Geometry check sheet. Reference: the model listing, model coordinates, mm. A direction names the side the tool comes from. Give positions to 0.01 mm unless a question says otherwise; leave off trailing zeros. Loops run counter-clockwise (first coordinate to the right, second up) from the corner with the lowest first, then second, coordinate; pieces in that order, holes last. Notation, with made-up numbers: (21.5, 76.25) -> (75.5, 76.25) arc R36 ccw to (75.5, 114.25) -> close; hole circle Ø9 at (-35, 72). An arc over 180 degrees is marked (long way). Answer as a JSON object with one key per item and string values.
from build123d import *

# Parameters (mm, degrees)
CROQUIS1_W              = 92
CROQUIS1_H              = 62
SALIENTE_EXTRUIR1_DEPTH = 18
CROQUIS2_W              = 87
CROQUIS2_H              = 57
CORTAR_EXTRUIR1_DEPTH   = 16
CROQUIS3_W              = 89
CROQUIS3_H              = 59
CROQUIS3_W_2            = 87
CROQUIS3_H_2            = 57
SALIENTE_EXTRUIR2_DEPTH = 2
CROQUIS4_W              = 2.5
CROQUIS4_H              = 14.150072655
CROQUIS4_H_2            = 13.999979608
CROQUIS4_H_3            = 17.009234147
CORTAR_EXTRUIR2_DEPTH   = 16
CROQUIS5_W              = 9.965409089
CROQUIS5_H              = 2.5
CROQUIS5_W_2            = 7.304626576
CROQUIS5_W_3            = 7.420347284
CROQUIS5_W_4            = 5
CORTAR_EXTRUIR3_DEPTH   = 5
CROQUIS7_R              = 2.5
CORTAR_EXTRUIR4_DEPTH   = 2
CROQUIS8_W              = 50.384335714
CROQUIS8_H              = 5
CORTAR_EXTRUIR5_DEPTH   = 2.5
CROQUIS9_W              = 56.605701511
CROQUIS9_H              = 16
CORTAR_EXTRUIR6_DEPTH   = 2.5


with BuildPart() as part:
    # Croquis1 → Saliente-Extruir1 (new body)
    with BuildSketch(Plane(origin=(0, 0, 0), x_dir=(1, 0, 0), z_dir=(0, 1, 0))):
        Rectangle(CROQUIS1_W, CROQUIS1_H)
    extrude(amount=SALIENTE_EXTRUIR1_DEPTH)

    # Croquis2 → Cortar-Extruir1 (cut)
    with BuildSketch(Plane(origin=(0, 18, 0), x_dir=(1, 0, 0), z_dir=(0, 1, 0))):
        Rectangle(CROQUIS2_W, CROQUIS2_H)
    extrude(amount=-CORTAR_EXTRUIR1_DEPTH, mode=Mode.SUBTRACT)

    # Croquis3 → Saliente-Extruir2 (add)
    with BuildSketch(Plane(origin=(0, 18, 0), x_dir=(1, 0, 0), z_dir=(0, 1, 0))):
        Rectangle(CROQUIS3_W, CROQUIS3_H)
        Rectangle(CROQUIS3_W_2, CROQUIS3_H_2, mode=Mode.SUBTRACT)
    extrude(amount=SALIENTE_EXTRUIR2_DEPTH)

    # Croquis4 → Cortar-Extruir2 (cut)
    with BuildSketch(Plane(origin=(0, 20, 0), x_dir=(1, 0, 0), z_dir=(0, 1, 0))):
        with Locations((-44.75, -18.476544129)):
            Rectangle(CROQUIS4_W, CROQUIS4_H)
        with Locations((-44.75, -0.477589339)):
            Rectangle(CROQUIS4_W, CROQUIS4_H_2)
        with Locations((-44.75, 18.601084438)):
            Rectangle(CROQUIS4_W, CROQUIS4_H_3)
    extrude(amount=-CORTAR_EXTRUIR2_DEPTH, mode=Mode.SUBTRACT)

    # Croquis5 → Cortar-Extruir3 (cut)
    with BuildSketch(Plane(origin=(0, 20, 0), x_dir=(1, 0, 0), z_dir=(0, 1, 0))):
        with Locations((31.175863948, -29.75)):
            Rectangle(CROQUIS5_W, CROQUIS5_H)
        with Locations((16.189846179, -29.75)):
            Rectangle(CROQUIS5_W_2, CROQUIS5_H)
        with Locations((2.577919336, -29.75)):
            Rectangle(CROQUIS5_W_3, CROQUIS5_H)
        with Locations((-11.725767222, -29.75)):
            Rectangle(CROQUIS5_W_4, CROQUIS5_H)
    extrude(amount=-CORTAR_EXTRUIR3_DEPTH, mode=Mode.SUBTRACT)

    # Croquis7 → Cortar-Extruir4 (cut)
    with BuildSketch(Plane.XZ):
        with Locations(Location((31, -16, 0), (0, 0, 270))):
            Circle(CROQUIS7_R)
        with Locations(Location((20.666666667, -16, 0), (0, 0, 270))):
            Circle(CROQUIS7_R)
        with Locations(Location((10.333333333, -16, 0), (0, 0, 270))):
            Circle(CROQUIS7_R)
        with Locations(Location((0, -16, 0), (0, 0, 270))):
            Circle(CROQUIS7_R)
        with Locations(Location((-10.333333333, -16, 0), (0, 0, 270))):
            Circle(CROQUIS7_R)
        with Locations(Location((-20.666666667, -16, 0), (0, 0, 270))):
            Circle(CROQUIS7_R)
        with Locations(Location((-31, -16, 0), (0, 0, 270))):
            Circle(CROQUIS7_R)
        with Locations(Location((20.666666667, -8, 0), (0, 0, 270))):
            Circle(CROQUIS7_R)
        with Locations(Location((10.333333333, -8, 0), (0, 0, 270))):
            Circle(CROQUIS7_R)
        with Locations(Location((0, -8, 0), (0, 0, 270))):
            Circle(CROQUIS7_R)
        with Locations(Location((-10.333333333, -8, 0), (0, 0, 270))):
            Circle(CROQUIS7_R)
        with Locations(Location((-20.666666667, -8, 0), (0, 0, 270))):
            Circle(CROQUIS7_R)
        with Locations(Location((-31, -8, 0), (0, 0, 270))):
            Circle(CROQUIS7_R)
        with Locations(Location((20.666666667, 0, 0), (0, 0, 270))):
            Circle(CROQUIS7_R)
        with Locations(Location((10.333333333, 0, 0), (0, 0, 270))):
            Circle(CROQUIS7_R)
        with Locations(Location((0, 0, 0), (0, 0, 270))):
            Circle(CROQUIS7_R)
        with Locations(Location((-10.333333333, 0, 0), (0, 0, 270))):
            Circle(CROQUIS7_R)
        with Locations(Location((-20.666666667, 0, 0), (0, 0, 270))):
            Circle(CROQUIS7_R)
        with Locations(Location((-31, 0, 0), (0, 0, 270))):
            Circle(CROQUIS7_R)
        with Locations(Location((20.666666667, 8, 0), (0, 0, 270))):
            Circle(CROQUIS7_R)
        with Locations(Location((10.333333333, 8, 0), (0, 0, 270))):
            Circle(CROQUIS7_R)
        with Locations(Location((0, 8, 0), (0, 0, 270))):
            Circle(CROQUIS7_R)
        with Locations(Location((-10.333333333, 8, 0), (0, 0, 270))):
            Circle(CROQUIS7_R)
        with Locations(Location((-20.666666667, 8, 0), (0, 0, 270))):
            Circle(CROQUIS7_R)
        with Locations(Location((-31, 8, 0), (0, 0, 270))):
            Circle(CROQUIS7_R)
        with Locations(Location((20.666666667, 16, 0), (0, 0, 270))):
            Circle(CROQUIS7_R)
        with Locations(Location((10.333333333, 16, 0), (0, 0, 270))):
            Circle(CROQUIS7_R)
        with Locations(Location((0, 16, 0), (0, 0, 270))):
            Circle(CROQUIS7_R)
        with Locations(Location((-10.333333333, 16, 0), (0, 0, 270))):
            Circle(CROQUIS7_R)
        with Locations(Location((-20.666666667, 16, 0), (0, 0, 270))):
            Circle(CROQUIS7_R)
        with Locations(Location((-31, 16, 0), (0, 0, 270))):
            Circle(CROQUIS7_R)
        with Locations(Location((31, -8, 0), (0, 0, 270))):
            Circle(CROQUIS7_R)
        with Locations(Location((31, 0, 0), (0, 0, 270))):
            Circle(CROQUIS7_R)
        with Locations(Location((31, 8, 0), (0, 0, 270))):
            Circle(CROQUIS7_R)
        with Locations(Location((31, 16, 0), (0, 0, 270))):
            Circle(CROQUIS7_R)
    extrude(amount=-CORTAR_EXTRUIR4_DEPTH, mode=Mode.SUBTRACT)

    # Croquis8 → Cortar-Extruir5 (cut)
    with BuildSketch(Plane.XY.offset(31)):
        with Locations((10.966400635, 17.5)):
            Rectangle(CROQUIS8_W, CROQUIS8_H)
    extrude(amount=-CORTAR_EXTRUIR5_DEPTH, mode=Mode.SUBTRACT)

    # Croquis9 → Cortar-Extruir6 (cut)
    with BuildSketch(Plane.ZY.offset(46)):
        with Locations((1.197149245, 12)):
            Rectangle(CROQUIS9_W, CROQUIS9_H)
    extrude(amount=-CORTAR_EXTRUIR6_DEPTH, mode=Mode.SUBTRACT)


solid = part.part
1) Section check D-D on y = 11.25. Record the cut outline in (x, z).
Geometry check:
{"outline": "(-46, -31) -> (46, -31) -> (46, 31) -> (-46, 31) -> (-46, 29.5) -> (-43.5, 29.5) -> (-43.5, 28.5) -> (43.5, 28.5) -> (43.5, -28.5) -> (-43.5, -28.5) -> (-43.5, -27.11) -> (-46, -27.11) -> close"}
2) Tool access check on faces 1 (the face through (-29, 19, 29.5)), 2 (the face through (-1, 11, 28.5)), 3 (the face through (-1, 19, -29.5)), 4 (the face through (-45, 11, 29.5)). Record the directions out of +Z, -Z, +X, -X, +Y, -Y that give a thin tool (end or side, any length) a straight path to the whole face; none if there is none.
Geometry check:
{"face 1": "+Z, +X, -X, +Y", "face 2": "+Y", "face 3": "-Z, +X, -X, +Y", "face 4": "-X, +Y"}
3) Material ranges on line 1 along Z through (x, y) = (1, 9.75); line 2 along X through (y, z) = (2.25, 18.5); line 3 along Y through (x, z) = (-30.5, -19.5), recorded low to high. Write a range as from..to.
Geometry check:
{"line 1": "z = -31..-28.5, 28.5..31", "line 2": "x = -46..-43.5, 43.5..46", "line 3": "y = 0..2"}
4) Draft check along Z on faces 5 (the face through (-1, 9, -31)), 6 (the face through (-45, 4, 1)), 7 (the face through (11, 15, 30)). Enter one of: pulls with the +Z half, pulls with the -Z half, needs draft (parallel to the pull), parting line crosses it, or undercut.
Geometry check:
{"face 5": "pulls with the -Z half", "face 6": "undercut", "face 7": "needs draft"}
5) Depth check by flat-ended pin: P1, Ø8, axis at x = 31, z = 0, coming from the +Y side; P2, Ø1, axis at x = -28.5, y = 19, coming from the +Z side; P3, Ø1.2, axis at x = -22.5, z = 30.5, coming from the +Y side. Enter the tip coordinate at first touch or a pass-through.
Geometry check:
{"P1": "stops at y = 2", "P2": "stops at z = 29.5", "P3": "stops at y = 18"}
6) Section check A-A on x = -31. Count the separate pieces of the cut face and the enclosed holes in it, plus the area to 3 significant figures.
Geometry check:
{"separate pieces": "6", "enclosed holes": "0", "area": "158 mm2"}
7) Section check B-B on y = 16.25. Record the cut outline in (x, z).
Geometry check:
{"outline": "(-46, -31) -> (46, -31) -> (46, 31) -> (36.16, 31) -> (36.16, 28.5) -> (43.5, 28.5) -> (43.5, -28.5) -> (-43.5, -28.5) -> (-43.5, -27.11) -> (-46, -27.11) -> close; (-46, 29.5) -> (-43.5, 29.5) -> (-43.5, 28.5) -> (-14.23, 28.5) -> (-14.23, 31) -> (-46, 31) -> close"}
